For this review, use the dimensioned drawing (mm, ordinates from the lowest corner) and the shaded views. Give positions to 0.01 mm unless a question says otherwise; leave off trailing zeros. Order: outer loops, then holes, each group sorted by start corner. A loop starts at its lowest first (then second) coordinate and runs counter-clockwise, first axis right, second up. Notation, with made-up numbers: (68.5, 80.5) - (123.5, 80.5) arc R17 ccw to (123.5, 105.5) - close; hole circle Ø3 at (1.25, 22). An arc over 180 degrees is marked (long way). One line per item, written item: value.
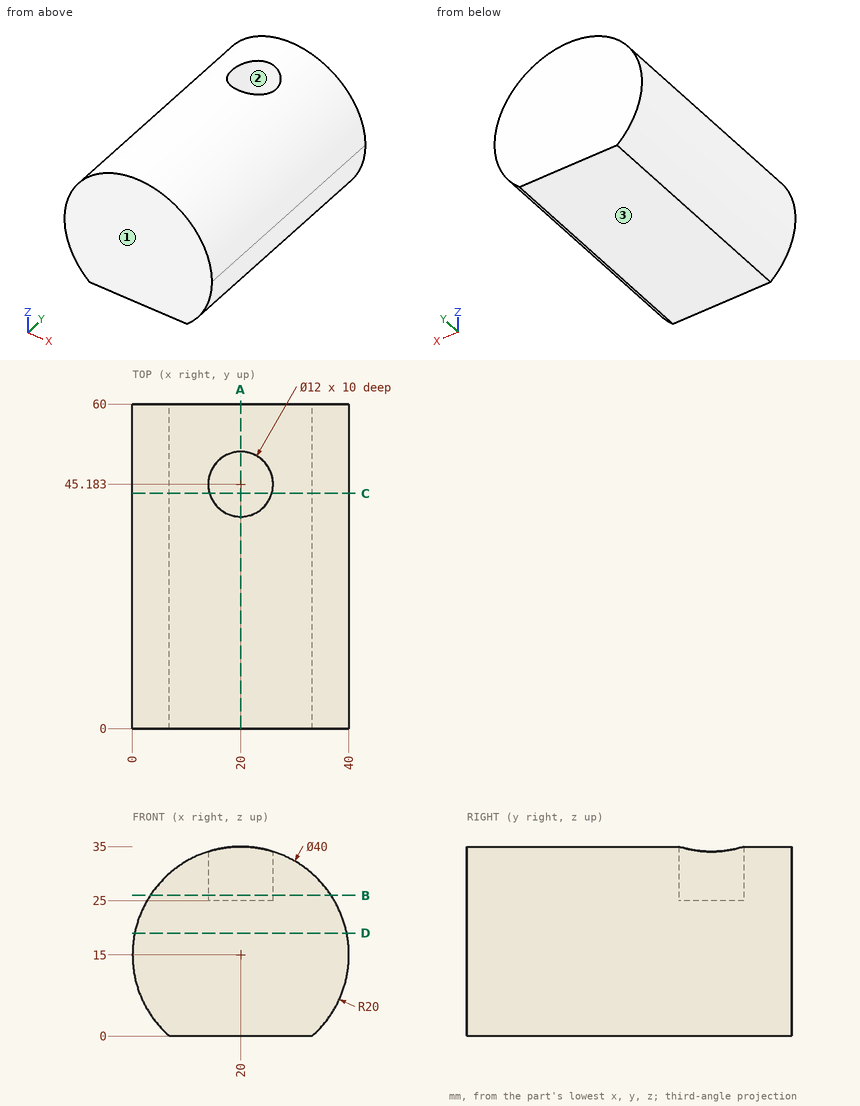
(1) Take a section at D-D (z = 19). Write out the cut boundary in (x, y).
Answers below:
outline: (0.4, 0) - (39.6, 0) - (39.6, 60) - (0.4, 60) - close
(2) Take a section at B-B (z = 26). Write out the cut boundary in (x, y), then the cut area to 3 significant figures.
Answers below:
outline: (3.3, 0) - (36.7, 0) - (36.7, 60) - (3.3, 60) - close; hole circle Ø12 at (20, 45.18)
area: 1,890 mm^2
(3) Draft analysis for pull direction Y (two halves, no side actions). For the marked faces 1, 2 and 3, state which applies: pulls with the +Y half, pulls with the -Y half, needs draft (parallel to the pull), parting line crosses it, or undercut.
Answers below:
face 1: pulls with the -Y half
face 2: undercut
face 3: needs draft
(4) Take a section at A-A (x = 20). Write out the cut boundary in (y, z).
Answers below:
outline: (0, 0) - (60, 0) - (60, 35) - (51.18, 35) - (51.18, 25) - (39.18, 25) - (39.18, 35) - (0, 35) - close
(5) Take a section at C-C (y = 43.5). Write out the cut boundary in (x, z).
Answers below:
outline: (6.77, 0) - (33.23, 0) arc R20 ccw to (25.76, 34.15) - (25.76, 25) - (14.24, 25) - (14.24, 34.15) arc R20 ccw to start
(6) For P1, Ø4, axis at y = 39, z = 17, coming from the -X side; P2, Ø4, axis at y = 7.5, z = 18, coming from the +X side (3 decimals); P3, Ø2, axis at x = 30, y = 21, coming from the +Z side; P4, Ø12, axis at y = 7.5, z = 27, coming from the +X side, all flat-tipped, find the tip position at first contact; note any pin that passes through.
Answers below:
P1: stops at x = 0
P2: stops at x = 39.975
P3: stops at z = 32.86
P4: stops at x = 39.08
(7) Wall thickness on line 1 (Y direction, x = 20, z = 30.25); line 2 (X direction, y = 36.5, z = 30); line 3 (X direction, y = 40, z = 29): over which ranges is each line inside the solid? List them lowest first. Write a range as from..to.
Answers below:
line 1: y = 0..39.18, 51.18..60
line 2: x = 6.77..33.23
line 3: x = 5.72..16.98, 23.02..34.28
